Answer from the drawing. Dimensions are ordinates in mm from the lowest x, y and z of the part. Coordinates: 2 decimals unless noted, no trailing zeros. Order: outer loops, then holes, each group sorted by start corner. A loop starts at its lowest first (then second) coordinate and runs counter-clockwise, first axis right, second up. Notation, with made-up numbers: (-13, 14) - (27, 14) arc R20 cw to (27, 19) - close; hole circle Ø11 at (50.5, 80.5). An arc over 180 degrees is marked (long way). One line per item, written item: value. Start each with the question number.
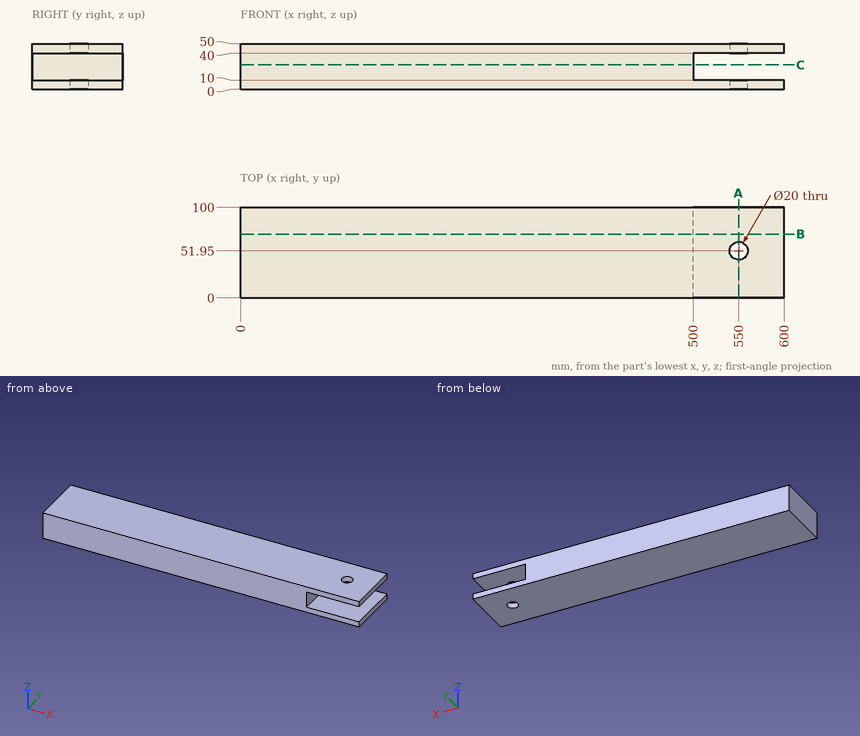
(1) Flat-ended cylindrical pins translate along their axes: pin 1 Ø15 at (y, z) = (42.5, 20) entering from +X; pin 2 Ø5 at (x, y) = (431.5, 73.5) entering from -Z. Find the tip coordinate at first contact, or state that the pin passes through.
(2) The part is cut by section C-C on z = 27. Determine the outline of the cut face in (x, y).
(3) The part is cut by section A-A on x = 550. Determine the outline of the cut face in (y, z).
(4) The part is cut by section B-B on y = 70.5. Determine the outline of the cut face in (x, z), plus the area to 3 significant figures.
(5) Consider probe 1 along Z at (x, y) = (530.5, 61.5); probe 2 along X at (y, z) = (92, 35); probe 3 along X at (y, z) = (56, 48). Determine where each line is inside the solid, lowest interval first.
Completed:
1. pin 1: stops at x = 500
1. pin 2: stops at z = 0
2. outline: (0, 0) - (500, 0) - (500, 100) - (0, 100) - close
3. outline: (0, 0) - (41.95, 0) - (41.95, 10) - (0, 10) - close; (0, 40) - (41.95, 40) - (41.95, 50) - (0, 50) - close; (61.95, 0) - (100, 0) - (100, 10) - (61.95, 10) - close; (61.95, 40) - (100, 40) - (100, 50) - (61.95, 50) - close
4. outline: (0, 0) - (600, 0) - (600, 10) - (500, 10) - (500, 40) - (600, 40) - (600, 50) - (0, 50) - close
4. area: 27,000 mm2
5. probe 1: z = 0 to 10, 40 to 50
5. probe 2: x = 0 to 500
5. probe 3: x = 0 to 540.86, 559.14 to 600
